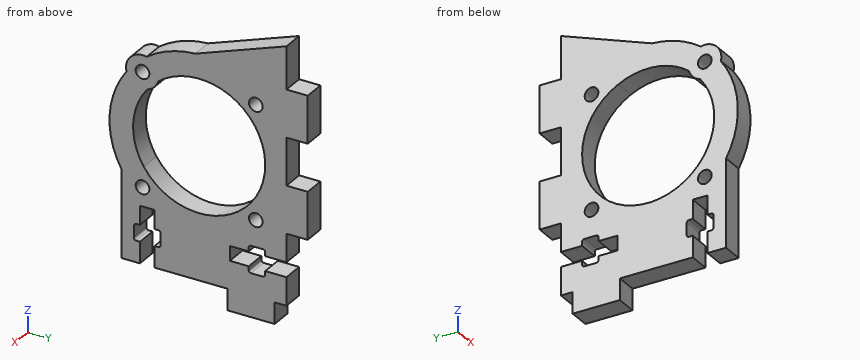
```python
from build123d import *

# Parameters (mm, degrees)
BOSS_EXTRUDE1_DEPTH  = 4.5
SKETCH2_W            = 9
SKETCH2_H            = 10
BOSS_EXTRUDE2_DEPTH  = 4.5
BOSS_EXTRUDE3_DEPTH  = 4.5
CUT_EXTRUDE1_DEPTH   = 65.507751472
SKETCH5_W            = 10
SKETCH5_H            = 4.5
BOSS_EXTRUDE4_DEPTH  = 4.5
CUT_EXTRUDE4_DEPTH   = 65.507751472
SKETCH12_R           = 14
SKETCH12_R_2         = 1.45
FANCUTOUT_DEPTH      = 65.507751472
BOSS_EXTRUDE7_DEPTH  = 4.5
SKETCH14_R           = 3.5
BOSS_EXTRUDE8_DEPTH  = 4.5
SKETCH15_R           = 1.45
CUT_EXTRUDE6_DEPTH   = 66.897647909
BOSS_EXTRUDE13_DEPTH = 4.5
BOSS_EXTRUDE15_DEPTH = 4.5


with BuildPart() as part:
    # Sketch1 → Boss-Extrude1 (new body)
    with BuildSketch(Plane(origin=(0, 0, 0), x_dir=(0, 0, -1), z_dir=(1, 0, 0))):
        Polygon((0, 0), (0, -35), (-54, 0), align=None)
    extrude(amount=BOSS_EXTRUDE1_DEPTH)

    # Sketch2 → Boss-Extrude2 (add, through all)
    with BuildSketch(Plane(origin=(4.5, 0, 0), x_dir=(0, 0, -1), z_dir=(1, 0, 0))):
        with Locations((0, -7.5)):
            Rectangle(SKETCH2_W, SKETCH2_H)
    extrude(amount=-BOSS_EXTRUDE2_DEPTH)

    # Sketch3 → Boss-Extrude3 (add, through all)
    with BuildSketch(Plane(origin=(4.5, 0, 0), x_dir=(0, 0, -1), z_dir=(1, 0, 0))):
        Polygon((0, -35), (-15, -35), (-54, 0), (0, -25), align=None)
    extrude(amount=-BOSS_EXTRUDE3_DEPTH)

    # Sketch4 → Cut-Extrude1 (cut, through all)
    with BuildSketch(Plane(origin=(4.5, 0, 0), x_dir=(0, 0, -1), z_dir=(1, 0, 0))):
        with BuildLine():
            Line((0, -31.05), (0, -27.95))
            Line((0, -27.95), (-4.5, -27.95))
            Line((-4.5, -27.95), (-4.5, -27.15))
            ThreePointArc((-4.5, -27.15), (-4.646446609, -26.796446609), (-5, -26.65))
            Line((-5, -26.65), (-7.5, -26.65))
            ThreePointArc((-7.5, -26.65), (-7.853553391, -26.796446609), (-8, -27.15))
            Line((-8, -27.15), (-8, -27.95))
            Line((-8, -27.95), (-12, -27.95))
            Line((-12, -27.95), (-12, -31.05))
            Line((-12, -31.05), (-8, -31.05))
            Line((-8, -31.05), (-8, -31.85))
            ThreePointArc((-8, -31.85), (-7.853553391, -32.203553391), (-7.5, -32.35))
            Line((-7.5, -32.35), (-5, -32.35))
            ThreePointArc((-5, -32.35), (-4.646446609, -32.203553391), (-4.5, -31.85))
            Line((-4.5, -31.85), (-4.5, -31.05))
            Line((-4.5, -31.05), (0, -31.05))
        make_face()
    extrude(amount=-CUT_EXTRUDE1_DEPTH, mode=Mode.SUBTRACT)

    # Sketch5 → Boss-Extrude4 (add, through all)
    with BuildSketch(Plane(origin=(4.5, 0, 0), x_dir=(0, 0, -1), z_dir=(1, 0, 0))):
        with Locations((-20, 2.25)):
            Rectangle(SKETCH5_W, SKETCH5_H)
        with Locations((-40, 2.25)):
            Rectangle(SKETCH5_W, SKETCH5_H)
    extrude(amount=-BOSS_EXTRUDE4_DEPTH)

    # Sketch11 → Cut-Extrude4 (cut, through all)
    with BuildSketch(Plane.ZY):
        with BuildLine():
            Line((5.95, -12), (9.05, -12))
            Line((9.05, -12), (9.05, -8))
            Line((9.05, -8), (9.85, -8))
            ThreePointArc((9.85, -8), (10.203553391, -7.853553391), (10.35, -7.5))
            Line((10.35, -7.5), (10.35, -5))
            ThreePointArc((10.35, -5), (10.203553391, -4.646446609), (9.85, -4.5))
            Line((9.85, -4.5), (9.05, -4.5))
            Line((9.05, -4.5), (9.05, 0))
            Line((9.05, 0), (5.95, 0))
            Line((5.95, 0), (5.95, -4.5))
            Line((5.95, -4.5), (5.15, -4.5))
            ThreePointArc((5.15, -4.5), (4.796446609, -4.646446609), (4.65, -5))
            Line((4.65, -5), (4.65, -7.5))
            ThreePointArc((4.65, -7.5), (4.796446609, -7.853553391), (5.15, -8))
            Line((5.15, -8), (5.95, -8))
            Line((5.95, -8), (5.95, -12))
        make_face()
    extrude(amount=-CUT_EXTRUDE4_DEPTH, mode=Mode.SUBTRACT)

    # Sketch12 → FanCutout (cut, through all)
    with BuildSketch(Plane.ZY):
        with Locations((28, -18.5)):
            Circle(SKETCH12_R)
        with Locations((16, -6.5)):
            Circle(SKETCH12_R_2)
        with Locations((40, -6.5)):
            Circle(SKETCH12_R_2)
        with Locations((16, -30.5)):
            Circle(SKETCH12_R_2)
    extrude(amount=-FANCUTOUT_DEPTH, mode=Mode.SUBTRACT)

    # Sketch13 → Boss-Extrude7 (add, through all)
    with BuildSketch(Plane.ZY):
        with BuildLine():
            Line((39.407071777, -10.383429697), (43.481025983, -7.484654589))
            ThreePointArc((43.481025983, -7.484654589), (41.102709954, -32.259323816), (16.241427695, -33.424341772))
            Line((16.241427695, -33.424341772), (19.335788828, -29.496883411))
            ThreePointArc((19.335788828, -29.496883411), (37.654628387, -28.638449127), (39.407071777, -10.383429697))
        make_face()
    extrude(amount=-BOSS_EXTRUDE7_DEPTH)

    # Sketch14 → Boss-Extrude8 (add, through all)
    with BuildSketch(Plane.ZY):
        with Locations((40, -30.5)):
            Circle(SKETCH14_R)
    extrude(amount=-BOSS_EXTRUDE8_DEPTH)

    # Sketch15 → Cut-Extrude6 (cut, through all)
    with BuildSketch(Plane.ZY):
        with Locations((40, -30.5)):
            Circle(SKETCH15_R)
    extrude(amount=-CUT_EXTRUDE6_DEPTH, mode=Mode.SUBTRACT)

    # Sketch24 → Boss-Extrude13 (add, through all)
    with BuildSketch(Plane.ZY):
        Polygon((15, -35), (20, -35), (16, -31.95), align=None)
    extrude(amount=-BOSS_EXTRUDE13_DEPTH)

    # Sketch25 → Boss-Extrude15 (add, through all)
    with BuildSketch(Plane.ZY):
        Polygon((54, 0), (46.982638315, -19.312060719), (44.28744936, -8.7163916), align=None)
    extrude(amount=-BOSS_EXTRUDE15_DEPTH)


solid = part.part
```
Geometry check sheet. Reference: the model listing, model coordinates, mm. Coordinates: 2 decimals unless noted, no trailing zeros. Write each loop counter-clockwise with the first axis right and the second up, starting at its lowest first coordinate (ties: lowest second). Pieces come first, ordered by that corner, then holes. Notation, with made-up numbers: M -17.5,1.25 L 14.5,1.25 A29 cw 14.5,31.25 Z; hole C 66.25,20.5 d10. An arc over 180 degrees is marked long. One line per item, written item: value. Start each with the question number.
(1) Sectioned sample at B-B, the plane y = -6.5. Enter the section's corners in (x, z), and give its area (3 significant figures).
(2) Sectioned sample at A-A, the plane z = 28. Enter the section's corners in (x, y).
(3) Sectioned sample at C-C, the plane z = 16. Enter the section's corners in (x, y), and give its area (4 significant figures).
(4) Depth check by flat-ended pin: pin 1 (2 mm diameter, centred on x = 1.5, z = 2, fed in from +Y); pin 2 (1.2 mm diameter, centred on x = 1.5, y = -1, fed in from -Z). Enter the tip coordinate at first touch or a pass-through.
(5) Scan lines: line 1 along Y through (x, z) = (1.05, 28); line 2 along Y through (x, z) = (3.3, 40); line 3 along Y through (x, z) = (2.1, 16). Record each from-to range of solid material in increasing order. Write a range as [from, to].
(6) Sectioned sample at D-D, the plane y = -18.5. Enter the section's corners in (x, z), and give its area (3 significant figures).
Filled sheet:
1. outline: M 0,-4.5 L 4.5,-4.5 L 4.5,4.65 L 0,4.65 Z; M 0,10.35 L 4.5,10.35 L 4.5,14.55 L 0,14.55 Z; M 0,17.45 L 4.5,17.45 L 4.5,20.79 L 0,20.79 Z; M 0,35.21 L 4.5,35.21 L 4.5,38.55 L 0,38.55 Z; M 0,41.45 L 4.5,41.45 L 4.5,51.64 L 0,51.64 Z
1. area: 136 mm²
2. outline: M 0,-37.5 L 4.5,-37.5 L 4.5,-32.5 L 0,-32.5 Z; M 0,-4.5 L 4.5,-4.5 L 4.5,0 L 0,0 Z
3. outline: M 0,-35 L 4.5,-35 L 4.5,-31.95 L 0,-31.95 Z; M 0,-29.05 L 4.5,-29.05 L 4.5,-25.71 L 0,-25.71 Z; M 0,-11.29 L 4.5,-11.29 L 4.5,-7.95 L 0,-7.95 Z; M 0,-5.05 L 4.5,-5.05 L 4.5,4.5 L 0,4.5 Z
3. area: 86.75 mm²
4. pin 1: y = 0
4. pin 2: z = 0
5. line 1: [-37.5, -32.5], [-4.5, 0]
5. line 2: [-34, -31.95], [-29.05, -25.71], [-11.29, -7.95], [-5.05, 4.5]
5. line 3: [-35, -31.95], [-29.05, -25.71], [-11.29, -7.95], [-5.05, 4.5]
6. outline: M 0,0 L 4.5,0 L 4.5,14 L 0,14 Z; M 0,42 L 4.5,42 L 4.5,47.28 L 0,47.28 Z
6. area: 86.7 mm²
